```python
from build123d import *

# Parameters (mm, degrees)
SKETCH1_R               = 7.9375
BOSS_EXTRUDE1_DEPTH     = 1.778
SKETCH2_R               = 4.7625
BOSS_EXTRUDE2_DEPTH     = 10.922
SKETCH4_R               = 3.96875
CUT_EXTRUDE3_DEPTH      = 1
CUT_EXTRUDE3_DEPTH_BACK = 13.7
SKETCH7_R               = 0.79375
CUT_EXTRUDE5_DEPTH      = 13.7


with BuildPart() as part:
    # Sketch1 → Boss-Extrude1 (new body)
    with BuildSketch(Plane(origin=(0, 0, 0), x_dir=(1, 0, 0), z_dir=(0, 1, 0))):
        Circle(SKETCH1_R)
    extrude(amount=BOSS_EXTRUDE1_DEPTH)

    # Sketch2 → Boss-Extrude2 (add)
    with BuildSketch(Plane(origin=(0, 1.778, 0), x_dir=(1, 0, 0), z_dir=(0, 1, 0))):
        Circle(SKETCH2_R)
    extrude(amount=BOSS_EXTRUDE2_DEPTH)

    # Sketch4 → Cut-Extrude3 (cut, two sides)
    with BuildSketch(Plane.XZ) as cut_extrude3_sk:
        Circle(SKETCH4_R)
    extrude(amount=CUT_EXTRUDE3_DEPTH, mode=Mode.SUBTRACT)
    extrude(cut_extrude3_sk.sketch, amount=-CUT_EXTRUDE3_DEPTH_BACK, mode=Mode.SUBTRACT)

    # Sketch7 → Cut-Extrude5 (cut, through all)
    with BuildSketch(Plane.XZ):
        with Locations((0, 6.604)):
            Circle(SKETCH7_R)
        with Locations((5.719231767, -3.302)):
            Circle(SKETCH7_R)
        with Locations((-5.719231767, -3.302)):
            Circle(SKETCH7_R)
    extrude(amount=-CUT_EXTRUDE5_DEPTH, mode=Mode.SUBTRACT)


solid = part.part
```
CAD build for the part. Positions are in the model's coordinates, mm. A direction names the side the tool comes from. Round coordinates to 2 decimals unless told otherwise and drop trailing zeros. Order: outer loops, then holes, each group sorted by start corner. A loop starts at its lowest first (then second) coordinate and runs counter-clockwise, first axis right, second up. Notation, with made-up numbers: (-15.5, 85) - (26.5, 85) arc R34 ccw to (26.5, 121) - close; hole circle Ø2 at (83.5, 1). An arc over 180 degrees is marked (long way). Answer as CSV lines item,"result". Start each with the question number.
1. Tool access for faces 4 (the face through (-5.891, 0.877, -4.077)), 5 (the face through (-3.78, 7.16, 2.9)): list every direction of +Z, -Z, +X, -X, +Y, -Y with a clear straight run to the whole face (end or side of a thin tool).
2. Pin check, flat tips, straight feed: pin 1 (2 mm diameter, centred on x = 0, z = 6.604, fed in from +Y); pin 2 (1 mm diameter, centred on y = 9, z = 0, fed in from -X); pin 3 (1.3 mm diameter, centred on x = -5.72, z = -3.3, fed in from -Y); pin 4 (2 mm diameter, centred on x = -1.5, y = 3.5, fed in from -Z). Stop position of each tip, or through.
3. Pull direction X, two halves, no side cores. Call faces 1 (the face through (5.1, 0.9, -3.8)), 2 (the face through (5, 1.778, 0)), 3 (the face through (-1.72, 0.88, 7.75)): +X half, -X half, draft (parallel to the pull), parting line (faces both ways), or undercut.
4. Saw through at C-C, the plane x = 6. Write the cut outline in (y, z), and give its area (3 significant figures).
5. Saw through at A-A, the plane x = 0. Write the cut outline in (y, z).
6. Saw through at B-B, the plane z = 0. Write the cut outline in (x, y).
7. Drill centre lines: L1, parallel to Z at x = 0, y = 5.25; L2, parallel to Y at x = -5.75, z = -2; L3, parallel to Z at x = 0.5, y = 7.25. Where is each one in solid material? Low to high. Write a range as [from, to].
8. Saw through at D-D, the plane y = 10.25. Write the cut outline in (x, z) (1 decimal).
Model answer:
1,face 4,"+Y, -Y"
1,face 5,"+Y"
2,pin 1,"stops at y = 1.78"
2,pin 2,"stops at x = -4.76"
2,pin 3,"passes through"
2,pin 4,"stops at z = -4.74"
3,face 1,"undercut"
3,face 2,"draft"
3,face 3,"parting line"
4,outline,"(0, -5.2) - (1.78, -5.2) - (1.78, -4.04) - (0, -4.04) - close; (0, -2.56) - (1.78, -2.56) - (1.78, 5.2) - (0, 5.2) - close"
4,area,"15.8 mm²"
5,outline,"(0, -7.94) - (1.78, -7.94) - (1.78, -4.76) - (12.7, -4.76) - (12.7, -3.97) - (0, -3.97) - close; (0, 3.97) - (12.7, 3.97) - (12.7, 4.76) - (1.78, 4.76) - (1.78, 5.81) - (0, 5.81) - close; (0, 7.4) - (1.78, 7.4) - (1.78, 7.94) - (0, 7.94) - close"
6,outline,"(-7.94, 0) - (-3.97, 0) - (-3.97, 12.7) - (-4.76, 12.7) - (-4.76, 1.78) - (-7.94, 1.78) - close; (3.97, 0) - (7.94, 0) - (7.94, 1.78) - (4.76, 1.78) - (4.76, 12.7) - (3.97, 12.7) - close"
7,L1,"z = [-4.76, -3.97], [3.97, 4.76]"
7,L2,"y = [0, 1.78]"
7,L3,"z = [-4.74, -3.94], [3.94, 4.74]"
8,outline,"circle Ø9.5 at (0, 0); hole circle Ø7.9 at (0, 0)"
